Answer from the drawing. Dimensions are ordinates in mm from the lowest x, y and z of the part. Coordinates: 2 decimals unless noted, no trailing zeros. Write each loop counter-clockwise with the first axis right and the second up, starting at its lowest first coordinate (ties: lowest second). Pieces come first, ordered by that corner, then holes.
(1) Section B-B on x = 6 is taken. Write down the section's boundary in (y, z), then the cut area to 3 significant figures.
(2) Section A-A on z = 4 is taken. Write down the section's boundary in (x, y).
(3) Section C-C on y = 2.75 is taken. Write down the section's boundary in (x, z).
(4) Given pin 1 (4 mm diameter, centred on y = 6.5, z = 5, fed in from +X), flat-ended and moving along its own axis, determine where the tip first touches the part or whether it passes through.
(5) Find the intervals of material crossed by probe 1 along Z at (x, y) = (3, 10.9); probe 2 along X at (y, z) = (1.25, 4.5); probe 3 along Y at (x, z) = (91, 3.5), in increasing order.
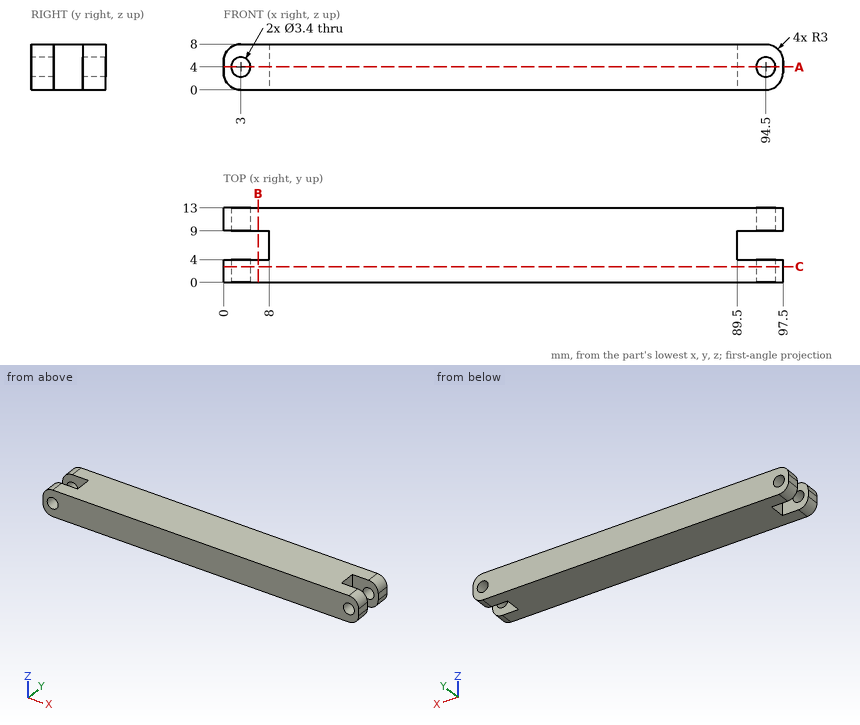
Response:
1. outline: (0, 0) - (4, 0) - (4, 8) - (0, 8) - close; (9, 0) - (13, 0) - (13, 8) - (9, 8) - close
1. area: 64.0 mm2
2. outline: (0, 0) - (1.3, 0) - (1.3, 4) - (0, 4) - close; (0, 9) - (1.3, 9) - (1.3, 13) - (0, 13) - close; (4.7, 0) - (92.8, 0) - (92.8, 4) - (89.5, 4) - (89.5, 9) - (92.8, 9) - (92.8, 13) - (4.7, 13) - (4.7, 9) - (8, 9) - (8, 4) - (4.7, 4) - close; (96.2, 0) - (97.5, 0) - (97.5, 4) - (96.2, 4) - close; (96.2, 9) - (97.5, 9) - (97.5, 13) - (96.2, 13) - close
3. outline: (0, 3) arc R3 ccw to (3, 0) - (94.5, 0) arc R3 ccw to (97.5, 3) - (97.5, 5) arc R3 ccw to (94.5, 8) - (3, 8) arc R3 ccw to (0, 5) - close; hole circle Ø3.4 at (3, 4); hole circle Ø3.4 at (94.5, 4)
4. pin 1: stops at x = 89.5
5. probe 1: z = 0 to 2.3, 5.7 to 8
5. probe 2: x = 0 to 1.38, 4.62 to 92.88, 96.12 to 97.5
5. probe 3: y = 0 to 4, 9 to 13
